from build123d import *

# Parameters (mm, degrees)
SKETCH1_R           = 3.935
SKETCH1_R_2         = 1.5
BOSS_EXTRUDE1_DEPTH = 3


with BuildPart() as part:
    # Sketch1 → Boss-Extrude1 (new body)
    with BuildSketch(Plane(origin=(0, 0, 0), x_dir=(1, 0, 0), z_dir=(0, 1, 0))):
        with BuildLine():
            Line((-5, -11.456439237), (-5, -30.5))
            ThreePointArc((-5, -30.5), (0, -35.5), (5, -30.5))
            Line((5, -30.5), (5, -11.456439237))
            ThreePointArc((5, -11.456439237), (0, 12.5), (-5, -11.456439237))
        make_face()
        with Locations(Location((0, 0, 0), (0, 0, 270))):
            Circle(SKETCH1_R, mode=Mode.SUBTRACT)
        with Locations(Location((0, 7, 0), (0, 0, 270))):
            Circle(SKETCH1_R_2, mode=Mode.SUBTRACT)
        with Locations(Location((0, -7, 0), (0, 0, 270))):
            Circle(SKETCH1_R_2, mode=Mode.SUBTRACT)
        with Locations(Location((0, -30.5, 0), (0, 0, 270))):
            Circle(SKETCH1_R_2, mode=Mode.SUBTRACT)
    extrude(amount=BOSS_EXTRUDE1_DEPTH)


solid = part.part
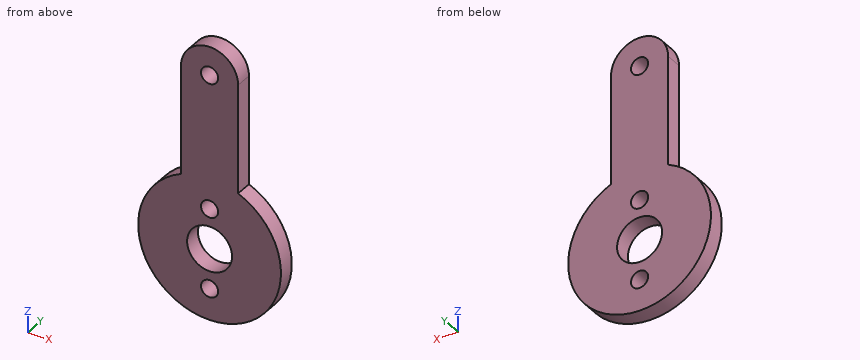
Check sheet for the modelled part. Datum: model origin and axes. Units: mm. Round coordinates to 2 decimals unless told otherwise and drop trailing zeros. Order: outer loops, then holes, each group sorted by start corner. A loop starts at its lowest first (then second) coordinate and runs counter-clockwise, first axis right, second up. Notation, with made-up numbers: M 31.25,-33.5 L 52.25,-33.5 A10 cw 52.25,-14.5 Z; hole C -10,86 d2. An arc over 180 degrees is marked long. One line per item, written item: value. Start each with the question number.
1. Scan lines: line 1 along X through (y, z) = (2.25, 28); line 2 along X through (y, z) = (1.75, 0) (3 decimals); line 3 along X through (y, z) = (1.95, -7). Record each from-to range of solid material in increasing order.
2. Section check C-C on y = 1.3. Enter the section's corners in (x, z) (3 decimals), and give its area (3 significant figures).
3. Section check B-B on x = 0. Enter the section's corners in (y, z) (3 decimals), and give its area (3 significant figures).
4. Gauge pin test, flat ends, axial feed: P1, Ø1, axis at x = 4.5, y = 1.5, coming from the -Z side; P2, Ø2, axis at x = 6.5, z = 26.5, coming from the +Y side. Record the tip position at first contact, or that the pin passes through.
5. Section check A-A on z = 0. Enter the section's corners in (x, y) (3 decimals).
6. Section check D-D on z = 7. Enter the section's corners in (x, y).
Results found:
1. line 1: -5 to 5
1. line 2: -12.5 to -3.935, 3.935 to 12.5
1. line 3: -10.36 to -1.5, 1.5 to 10.36
2. outline: M -5,11.456 A12.5 ccw long 5,11.456 L 5,30.5 A5 ccw -5,30.5 Z; hole C 0,0 d7.87; hole C 0,-7 d3; hole C 0,7 d3; hole C 0,30.5 d3
2. area: 644 mm^2
3. outline: M 0,-12.5 L 3,-12.5 L 3,-8.5 L 0,-8.5 Z; M 0,-5.5 L 3,-5.5 L 3,-3.935 L 0,-3.935 Z; M 0,3.935 L 3,3.935 L 3,5.5 L 0,5.5 Z; M 0,8.5 L 3,8.5 L 3,29 L 0,29 Z; M 0,32 L 3,32 L 3,35.5 L 0,35.5 Z
3. area: 93.4 mm^2
4. P1: z = -11.84
4. P2: through
5. outline: M -12.5,0 L -3.935,0 L -3.935,3 L -12.5,3 Z; M 3.935,0 L 12.5,0 L 12.5,3 L 3.935,3 Z
6. outline: M -10.36,0 L -1.5,0 L -1.5,3 L -10.36,3 Z; M 1.5,0 L 10.36,0 L 10.36,3 L 1.5,3 Z
